Geometry: final body of the model. Coordinates: model frame, mm. Face numbers are marked on the shaded views. A direction names the side the tool comes from. Coordinates: 2 decimals unless noted, no trailing zeros. Write each loop counter-clockwise with the first axis right and the second up, starting at its lowest first coordinate (ties: lowest second). Pieces come first, ordered by that corner, then holes.
from build123d import *

# Parameters (mm, degrees)
CUT_EXTRUDE_9_DEPTH         = 191.91883092
CUT_EXTRUDE_9_DEPTH_BACK    = 191.91883092
SKETCH_6_W                  = 50
SKETCH_6_H                  = 5.5
CUT_EXTRUDE_4_DEPTH         = 5
CUT_EXTRUDE_10_DEPTH        = 191.91883092
CUT_EXTRUDE_10_DEPTH_BACK   = 191.91883092
SKETCH_16_R                 = 5
HOLE_WIZARD_0_15_32_1_D     = 32
HOLE_WIZARD_0_15_32_1_DEPTH = 50
HOLE_WIZARD_0_15_32_1_TIP   = 9.613769904
CHAMFER_3_SIZE              = 2
CHAMFER_4_SIZE              = 2.5
CHAMFER_5_SIZE              = 2


with BuildPart() as part:
    # Эскиз1 → Повернуть1 (revolve)
    with BuildSketch(Plane.XY, mode=Mode.PRIVATE) as revolve_1_sk:
        Polygon((0, 16), (0, 20), (55, 20), (55, 30), (135, 30), (135, 45), (180, 45), (180, 16), align=None)
    revolve(revolve_1_sk.sketch.rotate(Axis((0, 0, 0), (-1, 0, 0)), 90), axis=Axis((0, 0, 0), (-1, 0, 0)))

    # Эскиз15 → Вырез-Вытянуть9 (cut, two sides: drawn at the far end of the back side and taken through both)
    with BuildSketch(Plane(origin=(180, 0, 0), x_dir=(0, 0, -1), z_dir=(1, 0, 0)).offset(-CUT_EXTRUDE_9_DEPTH_BACK)):
        with BuildLine():
            Line((-35, -28.284271247), (-35, 28.284271247))
            ThreePointArc((-35, 28.284271247), (-45, 0), (-35, -28.284271247))
        make_face()
    extrude(amount=CUT_EXTRUDE_9_DEPTH + CUT_EXTRUDE_9_DEPTH_BACK, mode=Mode.SUBTRACT)

    # Эскиз6 → Вырез-Вытянуть4 (cut, symmetric)
    with BuildSketch(Plane.XY):
        with Locations((95, 27.25)):
            Rectangle(SKETCH_6_W, SKETCH_6_H)
    extrude(amount=CUT_EXTRUDE_4_DEPTH, both=True, mode=Mode.SUBTRACT)

    # Эскиз16 → Вырез-Вытянуть10 (cut, two sides: drawn at the far end of the back side and taken through both)
    with BuildSketch(Plane(origin=(0, 0, 0), x_dir=(1, 0, 0), z_dir=(0, 1, 0)).offset(-CUT_EXTRUDE_10_DEPTH_BACK)):
        with Locations(Location((25, 0, 0), (0, 0, 270))):
            Circle(SKETCH_16_R)
    extrude(amount=CUT_EXTRUDE_10_DEPTH + CUT_EXTRUDE_10_DEPTH_BACK, mode=Mode.SUBTRACT)

    # Диаметр отверстия Ø0.15 (32)1
    with Locations(Plane.XY.offset(35)):
        with Locations((157.5, 0)):
            Hole(HOLE_WIZARD_0_15_32_1_D / 2, depth=HOLE_WIZARD_0_15_32_1_DEPTH)
            with Locations((0, 0, -(HOLE_WIZARD_0_15_32_1_DEPTH + HOLE_WIZARD_0_15_32_1_TIP / 2))):  # 118° drill point
                Cone(0, HOLE_WIZARD_0_15_32_1_D / 2, HOLE_WIZARD_0_15_32_1_TIP, mode=Mode.SUBTRACT)

    # Фаска3
    chamfer_3_edges = [part.edges().sort_by_distance(p)[0] for p in [
        (0, 0, 16),
        (0, 0, 20),
    ]]
    chamfer(chamfer_3_edges, length=CHAMFER_3_SIZE - 0.0001)  # a hair under: the kernel refuses the full size

    # Фаска4
    chamfer_4_edges = [part.edges().sort_by_distance(p)[0] for p in [
        (180, 0, -45),
        (135, 0, -45),
    ]]
    chamfer(chamfer_4_edges, length=CHAMFER_4_SIZE)

    # Фаска5
    chamfer_5_edges = [part.edges().sort_by_distance(p)[0] for p in [
        (55, 0, 30),
    ]]
    chamfer(chamfer_5_edges, length=CHAMFER_5_SIZE)


solid = part.part
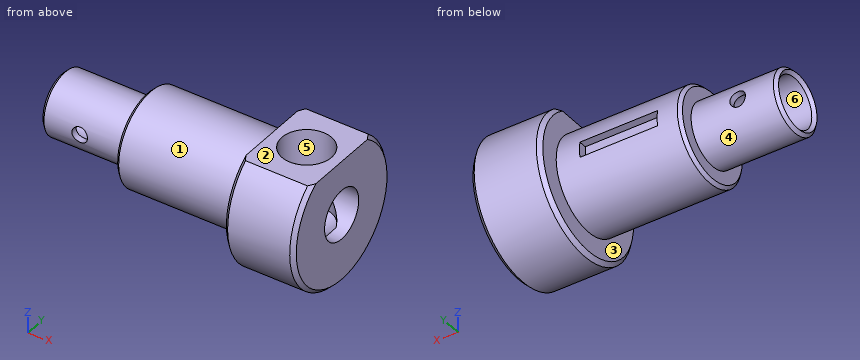
Item 1: Pin query (flat end, axial travel): pin 1 (16 mm diameter, centred on x = 25, z = 0, fed in from +Y); pin 2 (10 mm diameter, centred on y = -15.5, z = 15.5, fed in from -X); pin 3 (10 mm diameter, centred on y = -22, z = 26.5, fed in from -X); pin 4 (1.6 mm diameter, centred on y = 26.5, z = -2, fed in from -X). Return the tip coordinate at first contact, or that it passes through.
Derived:
pin 1: stops at y = 20
pin 2: stops at x = 0
pin 3: stops at x = 56.44
pin 4: stops at x = 55
Item 2: Material intervals for probe 1 along Z at (x, y) = (11, 0.5); probe 2 along Y at (x, z) = (167, 0); probe 3 along X at (y, z) = (22.5, 20.5), sorted ascending.
Derived:
probe 1: z = -19.99 to -15.99, 15.99 to 19.99
probe 2: y = -45 to -16, 16 to 45
probe 3: x = 135 to 180
Item 3: Set-up query: the marked faces 1 and 2. Return all of +Z, -Z, +X, -X, +Y, -Y with unobstructed straight access to the full face (end or side cutting, diameter ignored); none if empty.
Derived:
face 1: -X
face 2: +Z, +X, -X, +Y, -Y
Item 4: Section B-B, the plane x = 67.5. Output: boundary loops of the cut face in (y, z), plus the area to 3 significant figures.
Derived:
outline: circle Ø60 at (0, 0); hole circle Ø32 at (0, 0)
area: 2,020 mm2
Item 5: Pull-direction query (Y, two-part tool) for the marked faces 3, 4, 5 and 6; classes: released by +Y, released by -Y, zero draft, split by the parting line, or undercut.
Derived:
face 3: zero draft
face 4: split by the parting line
face 5: undercut
face 6: undercut
Item 6: Section C-C, the plane z = 2. State how many separate pieces and enclosed holes the cut face has, plus the area to 3 significant figures.
Derived:
separate pieces: 4
enclosed holes: 0
area: 4,940 mm2
Item 7: Section A-A, the plane x = 25. Output: boundary loops of the cut face in (y, z), plus the area to 3 significant figures.
Derived:
outline: (-19.36, -5) arc R20 ccw to (19.36, -5) - (15.2, -5) arc R16 cw to (-15.2, -5) - close; (-19.36, 5) - (-15.2, 5) arc R16 cw to (15.2, 5) - (19.36, 5) arc R20 ccw to start
area: 371 mm2
